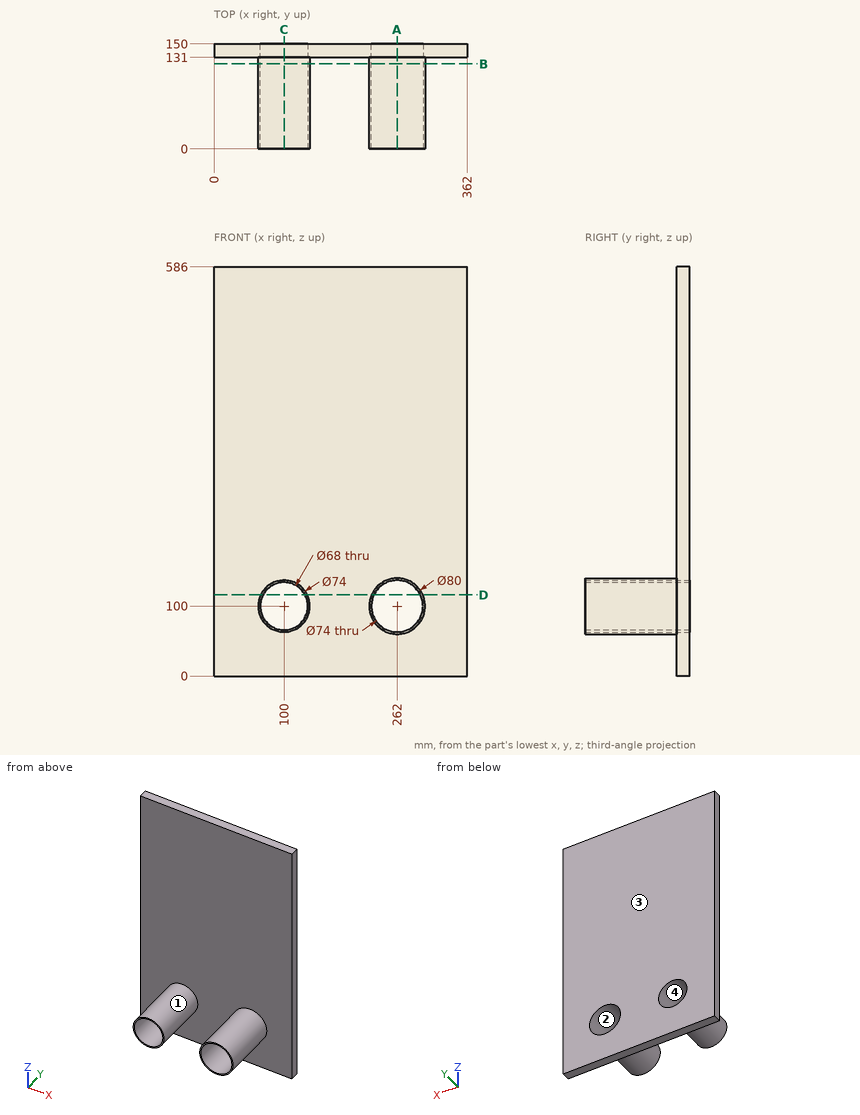
Geometry: see drawing. Coordinates: mm, zero at the bounding-box minimum. A direction names the side the tool comes from. Give positions to 0.01 mm unless a question says otherwise; leave off trailing zeros. Order: outer loops, then holes, each group sorted by start corner. A loop starts at its lowest first (then second) coordinate and runs counter-clockwise, first axis right, second up. Notation, with made-up numbers: (-18, 7.5) - (26, 7.5) arc R4 ccw to (26, 12.5) - close; hole circle Ø1 at (32.5, 37). An arc over 180 degrees is marked (long way). Write each question's results on one line, items separated by ' | '.
Item 1: Section B-B (y = 121.5). Return loops of the section in (x, z).
A:
outline: circle Ø74 at (100, 100); circle Ø80 at (262, 100); hole circle Ø68 at (100, 100); hole circle Ø74 at (262, 100)
Item 2: Section D-D (z = 116). Return loops of the section in (x, y).
A:
outline: (0, 131) - (66.64, 131) - (66.64, 0) - (70, 0) - (70, 150) - (0, 150) - close; (130, 0) - (133.36, 0) - (133.36, 131) - (225.34, 131) - (225.34, 0) - (228.64, 0) - (228.64, 150) - (130, 150) - close; (295.36, 0) - (298.66, 0) - (298.66, 131) - (362, 131) - (362, 150) - (295.36, 150) - close
Item 3: Contact query for flat-ended pins moving along their axis: pin 1 Ø5 at (x, y) = (243.5, 28.5) entering from -Z; pin 2 Ø6 at (x, y) = (249, 54) entering from +Z; pin 3 Ø5 at (x, z) = (106, 313) entering from -Y. Output: stop coordinate, or through.
A:
pin 1: stops at z = 63.34 | pin 2: stops at z = 138.73 | pin 3: stops at y = 131
Item 4: Material intervals for line 1 along X through (y, z) = (124, 92); line 2 along Z through (x, y) = (100, 85); line 3 along Z through (x, y) = (262, 103.5), sorted ascending.
A:
line 1: x = 63.88 to 66.95, 133.05 to 136.12, 222.81 to 225.88, 298.12 to 301.19 | line 2: z = 63 to 66, 134 to 137 | line 3: z = 60 to 63, 137 to 140
Item 5: Section C-C (x = 100). Return loops of the section in (y, z).
A:
outline: (0, 63) - (131, 63) - (131, 0) - (150, 0) - (150, 66) - (0, 66) - close; (0, 134) - (150, 134) - (150, 586) - (131, 586) - (131, 137) - (0, 137) - close
Item 6: Access query for the marked faces 1 and 2. Directions: +Z, -Z, +X, -X, +Y, -Y. A direction counts if a zero-diameter tool reaches every point of the face in a straight line with its end or side. Return the directions, or none.
A:
face 1: -Y | face 2: +Y, -Y
Item 7: Section A-A (x = 262). Return loops of the section in (y, z), and give its area (3 significant figures).
A:
outline: (0, 60) - (131, 60) - (131, 0) - (150, 0) - (150, 63) - (0, 63) - close; (0, 137) - (150, 137) - (150, 586) - (131, 586) - (131, 140) - (0, 140) - close | area: 10,500 mm^2
Item 8: Draft query along X for the marked faces 3 and 4. Return one class per face: released by +X, released by -X, zero draft, split by the parting line, or undercut.
A:
face 3: zero draft | face 4: undercut
